```python
from build123d import *

# Parameters (mm, degrees)
F0_W     = 12.7
F0_H     = 19.05
F1_DEPTH = 152.4
F2_W     = 19.05
F2_H     = 10.359494
F3_DEPTH = 25.4
F5_D     = 6.4008


with BuildPart() as f1:
    # F0 (on Right) → F1 (new body)
    with BuildSketch(Plane.YZ):
        with Locations((2.279275, -0.169806)):
            Rectangle(F0_W, F0_H)
    extrude(amount=F1_DEPTH)

    # F2 (on face) → F3 (cut)
    with BuildSketch(Plane.XZ.offset(4.070725)):
        with Locations((22.225, 4.175447)):
            Rectangle(F2_W, F2_H)
    extrude(amount=-F3_DEPTH, mode=Mode.SUBTRACT)

    # F5 (through all)
    with Locations(Plane.XZ.offset(4.070725)):
        with Locations((137.973741, 0)):
            Hole(F5_D / 2)


solid = f1.part
```
Work out the finished part from the listing and answer in its coordinate system (mm). A direction names the side the tool comes from. Give positions to 0.01 mm unless a question says otherwise; leave off trailing zeros. Loops run counter-clockwise (first coordinate to the right, second up) from the corner with the lowest first, then second, coordinate; pieces in that order, holes last. Notation, with made-up numbers: (82, -14.5) -> (116, -14.5) arc R19 cw to (116, 17.5) -> close; hole circle Ø5 at (20, 70.25). An arc over 180 degrees is marked (long way). Write item = value, one per line. Start each with the question number.
(1) The mould has two halves that part along Z. Classify faces 1 (the flat face through (6, 2, 9.355)), 2 (the cylindrical face through (141.17, 2.37, 0.14)), 3 (the flat face through (31.75, 2, 4)), 4 (the flat face through (75, 2, -9.695)): +Z half, -Z half, draft (parallel to the pull), parting line (faces both ways), or undercut.
(2) Find section A-A on y = 6.75. Give the vertices of the cut face in (x, z), and give its area (3 significant figures).
(3) Which of the six approach directions +Z, -Z, +X, -X, +Y, -Y give full straight-line access (tool end or side, diameter ignored) to faces 5 (the flat face through (22, 2, -1.004)), 6 (the flat face through (91, 2, 9.355))?
(4) Find the intervals of material crossed by probe 1 along X at (y, z) = (-1.75, 6.5); probe 2 along X at (y, z) = (1.25, -2); probe 3 along Z at (x, y) = (21, 6.75), in increasing order. Write a range as from..to.
(5) Find section C-C on x = 136.5. Give the vertices of the cut face in (y, z), and give its area (3 significant figures).
(6) Find section B-B on z = 1.25. Give the vertices of the cut face in (x, y).
(7) Find section D-D on x = 26.5. Give the vertices of the cut face in (y, z).
From the geometry:
q1.face_1 = +Z half
q1.face_2 = undercut
q1.face_3 = draft
q1.face_4 = -Z half
q2.outline = (0, -9.69) -> (152.4, -9.69) -> (152.4, 9.36) -> (31.75, 9.36) -> (31.75, -1) -> (12.7, -1) -> (12.7, 9.36) -> (0, 9.36) -> close; hole circle Ø6.4 at (137.97, 0)
q2.area = 2,670 mm^2
q3.face_5 = +Z, +Y, -Y
q3.face_6 = +Z, +X, -X, +Y, -Y
q4.probe_1 = 0..12.7, 31.75..152.4
q4.probe_2 = 0..135.48, 140.47..152.4
q4.probe_3 = -9.69..-1
q5.outline = (-4.07, -9.69) -> (8.63, -9.69) -> (8.63, -2.84) -> (-4.07, -2.84) -> close; (-4.07, 2.84) -> (8.63, 2.84) -> (8.63, 9.36) -> (-4.07, 9.36) -> close
q5.area = 170 mm^2
q6.outline = (0, -4.07) -> (12.7, -4.07) -> (12.7, 8.63) -> (0, 8.63) -> close; (31.75, -4.07) -> (135.03, -4.07) -> (135.03, 8.63) -> (31.75, 8.63) -> close; (140.92, -4.07) -> (152.4, -4.07) -> (152.4, 8.63) -> (140.92, 8.63) -> close
q7.outline = (-4.07, -9.69) -> (8.63, -9.69) -> (8.63, -1) -> (-4.07, -1) -> close
